Check sheet for the modelled part. Datum: model origin and axes. Units: mm. A direction names the side the tool comes from. Coordinates: 2 decimals unless noted, no trailing zeros. Order: outer loops, then holes, each group sorted by start corner. A loop starts at its lowest first (then second) coordinate and runs counter-clockwise, first axis right, second up.
from build123d import *

# Parameters (mm, degrees)
F0_W           = 215
F0_H           = 115
F1_DEPTH       = 30
F3_T           = -2
F4_W           = 16
F4_H           = 111
F2_R           = 25
F5_DEPTH       = 2
F9_D           = 3.2
F9_DEPTH       = 5
F9_TIP         = 0.9613769904
F9_ON_F7_D     = 3.2
F9_ON_F7_DEPTH = 5
F9_ON_F7_TIP   = 0.9613769904
F9_ON_F8_D     = 3.2
F9_ON_F8_DEPTH = 5
F9_ON_F8_TIP   = 0.9613769904


with BuildPart() as f1:
    # F0 (on Top) → F1 (new body)
    with BuildSketch(Plane.XY):
        Rectangle(F0_W, F0_H)
    extrude(amount=F1_DEPTH)

    # F3
    f3_openings = [f1.faces().sort_by_distance(p)[0] for p in [
        (-107.5, 0, 15),
    ]]
    offset(amount=F3_T, openings=f3_openings)

    # F4 (on face) + F2 (on face) → F5 (cut, through all)
    with BuildSketch(Plane.XY.offset(30)):
        with Locations((-99.5, 0)):
            Rectangle(F4_W, F4_H)
    with BuildSketch(Plane.XY.offset(30)):
        with Locations((60.05, 20.8)):
            Circle(F2_R)
    extrude(amount=-F5_DEPTH, mode=Mode.SUBTRACT)

    # F9
    with Locations(Plane(origin=(0, 0, 0), x_dir=(1, 0, 0), z_dir=(0, 0, -1))):
        with Locations((-75, 25), (75, -25), (-75, -25), (75, 25)):
            Hole(F9_D / 2, depth=F9_DEPTH)
            with Locations((0, 0, -(F9_DEPTH + F9_TIP / 2))):  # 118° drill point
                Cone(0, F9_D / 2, F9_TIP, mode=Mode.SUBTRACT)

    # F9 on F7
    with Locations(Plane.XZ.offset(57.5)):
        with Locations((-75, 12.5), (75, 12.5)):
            Hole(F9_ON_F7_D / 2, depth=F9_ON_F7_DEPTH)
            with Locations((0, 0, -(F9_ON_F7_DEPTH + F9_ON_F7_TIP / 2))):  # 118° drill point
                Cone(0, F9_ON_F7_D / 2, F9_ON_F7_TIP, mode=Mode.SUBTRACT)

    # F9 on F8
    with Locations(Plane(origin=(0, 57.5, 0), x_dir=(-1, 0, 0), z_dir=(0, 1, 0))):
        with Locations((-75, 12.5), (75, 12.5)):
            Hole(F9_ON_F8_D / 2, depth=F9_ON_F8_DEPTH)
            with Locations((0, 0, -(F9_ON_F8_DEPTH + F9_ON_F8_TIP / 2))):  # 118° drill point
                Cone(0, F9_ON_F8_D / 2, F9_ON_F8_TIP, mode=Mode.SUBTRACT)


solid = f1.part
(1) Tool access check on faces 1 (the flat face through (-2, -57.5, 15)), 2 (the cylindrical face through (83.9, 28.3, 29)), 3 (the flat face through (105.5, -1, 15)). Record the directions out of +Z, -Z, +X, -X, +Y, -Y that give a thin tool (end or side, any length) a straight path to the whole face; none if there is none.
Filled in:
face 1: +Z, -Z, +X, -X, -Y
face 2: +Z
face 3: -X
(2) Cross-section at C-C (x = -69). Enter the section's corners in (y, z), and give its area (3 significant figures).
Filled in:
outline: (-57.5, 0) - (57.5, 0) - (57.5, 30) - (-57.5, 30) - close; hole (-55.5, 2) - (55.5, 2) - (55.5, 28) - (-55.5, 28) - close
area: 564 mm2
(3) Cross-section at A-A (y = 20.8). Enter the section's corners in (x, z).
Filled in:
outline: (-107.5, 0) - (107.5, 0) - (107.5, 30) - (85.05, 30) - (85.05, 28) - (105.5, 28) - (105.5, 2) - (-107.5, 2) - close; (-91.5, 28) - (35.05, 28) - (35.05, 30) - (-91.5, 30) - close
(4) Thickness scan on probe 1 along Y at (x, z) = (-75, 1.5); probe 2 along Y at (x, z) = (-69, 15.5); probe 3 along Z at (x, y) = (69, 49.5). Record the ranges inside material, lowest first.
Filled in:
probe 1: y = -57.5 to -26.6, -23.4 to 23.4, 26.6 to 57.5
probe 2: y = -57.5 to -55.5, 55.5 to 57.5
probe 3: z = 0 to 2, 28 to 30
(5) Release check for a two-part mould opening along Y. For faces 4 (the flat face through (-2, 57.5, 15)), 5 (the flat face through (-2, 55.5, 16)), 6 (the flat face through (107.5, -1, 15)) record: +Y half, -Y half, draft (parallel to the pull), parting line (faces both ways), or undercut.
Filled in:
face 4: +Y half
face 5: undercut
face 6: draft
(6) Cross-section at B-B (z = 25.25). Enter the section's corners in (x, y).
Filled in:
outline: (-107.5, -57.5) - (107.5, -57.5) - (107.5, 57.5) - (-107.5, 57.5) - (-107.5, 55.5) - (105.5, 55.5) - (105.5, -55.5) - (-107.5, -55.5) - close
(7) Go/stop test with flat-tipped pins: P1, Ø3.5, axis at x = 75, y = 25, coming from the +Z side; P2, Ø3, axis at y = 33, z = 21, coming from the -X side; P3, Ø1, axis at y = 4.5, z = 29, coming from the -X side. Record where each tip stops, or that it passes through.
Filled in:
P1: stops at z = 2
P2: stops at x = 105.5
P3: stops at x = -91.5
(8) Cross-section at D-D (y = -46). Enter the section's corners in (x, z).
Filled in:
outline: (-107.5, 0) - (107.5, 0) - (107.5, 30) - (-91.5, 30) - (-91.5, 28) - (105.5, 28) - (105.5, 2) - (-107.5, 2) - close
